Could you check a few things on this drawing? It's one solid part, dimensions in mm from its lowest x, y, z. A direction names the side the tool comes from. Coordinates: 2 decimals unless noted, no trailing zeros. Write each loop counter-clockwise with the first axis right and the second up, starting at its lowest first coordinate (ties: lowest second). Pieces come first, ordered by that corner, then holes. Notation, with made-up numbers: (-15, -16.75) - (6, -16.75) arc R29 ccw to (6, 14.25) - close; hole circle Ø4 at (-37.75, 9). An arc over 180 degrees is marked (long way). Use one line per item in the form item = value. Start each with the question number.
(1) Thinking about a two-plate mould opening in X: for the marked faces 3, 4 and 5, which applies, pulls with the +X half, pulls with the -X half, needs draft (parallel to the pull), parting line crosses it, or undercut?
(2) For pin 1 Ø2.5 at (y, z) = (5, 15) entering from -X; pin 2 Ø2 at (x, z) = (22.5, 7.5) entering from -Y, each with a flat end and sliding along its axis, tell me the tip position at first contact or that it passes through.
(3) If I drill on probe 1 along Z at (x, y) = (25.25, 5); probe 2 along X at (y, z) = (3.75, 7.5); probe 3 along Y at (x, z) = (15, 10.5), over which ranges is the centre line in solid material (lowest first)? Write a range as from..to.
(4) If we section it at D-D on z = 5.5: Please give me the cut outline in (x, y), then the cut area to 3 significant figures.
(5) If we section it at C-C on y = 5: Give the number of separate pieces and of enclosed holes in the cut face, then the cut area to 3 significant figures.
(6) On a 3-axis mill with a long thin cutter (end or side, diameter ignored), from which of +Z, -Z, +X, -X, +Y, -Y can I reach the whole of each face in a straight line? I mean the marked faces 1 and 2. Say none if no direction works.
(7) If we section it at B-B on x = 24.75: Please give me the cut outline in (y, z).
(8) If we section it at A-A on y = 15: Please give me the cut outline in (x, z).
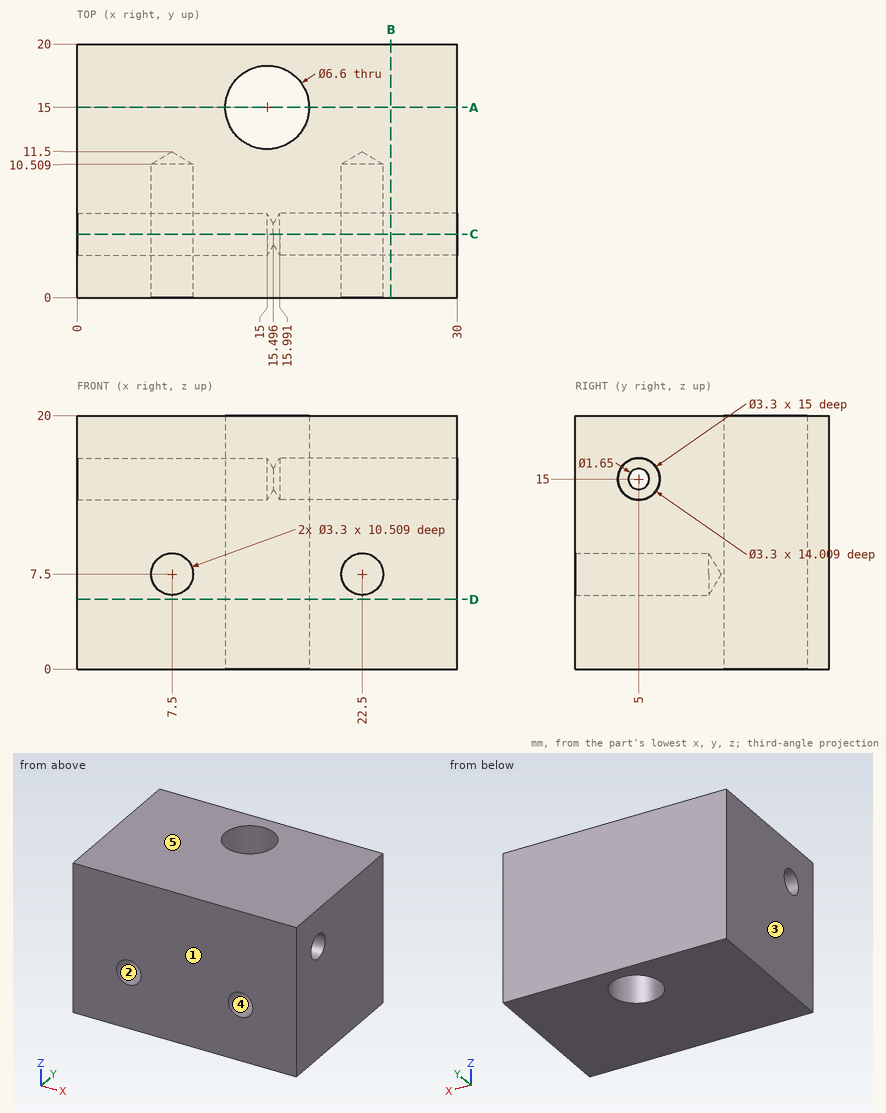
Reported:
q1.face_3 = pulls with the -X half
q1.face_4 = undercut
q1.face_5 = needs draft
q2.pin_1 = 15.24
q2.pin_2 = 10.9
q3.probe_1 = 0..13.35, 16.65..20
q3.probe_2 = 0..5.85, 9.15..20.85, 24.15..30
q3.probe_3 = 0..11.7, 18.3..20
q4.outline = (0, 0) - (30, 0) - (30, 20) - (0, 20) - close; hole circle Ø6.6 at (15, 15)
q4.area = 566 mm2
q5.separate_pieces = 2
q5.enclosed_holes = 2
q5.area = 485 mm2
q6.face_1 = +Z, -Z, +X, -X, -Y
q6.face_2 = -Y
q7.outline = (0, 0) - (20, 0) - (20, 20) - (0, 20) - close; hole circle Ø3.3 at (5, 15)
q8.outline = (0, 0) - (11.7, 0) - (11.7, 20) - (0, 20) - close; (18.3, 0) - (30, 0) - (30, 20) - (18.3, 20) - close
